Here's how the part is built. I have some questions about the finished solid (model axes, mm). Face numbers are marked on the shaded views. Coordinates: 2 decimals unless noted, no trailing zeros. Loops run counter-clockwise (first coordinate to the right, second up) from the corner with the lowest first, then second, coordinate; pieces in that order, holes last. Notation, with made-up numbers: M 70.5,-8.75 L 122.5,-8.75 A35 cw 122.5,30.25 Z; hole C 77,46.5 d10. An arc over 180 degrees is marked long. Use CSV: the item, a comma, the result in double quotes. Start each with the question number.
Q1. If we section it at B-B (x = -2.5): Please give me the cut outline in (y, z) (3 decimals), and give its area (3 significant figures).
Q2. Please list where these lines run through material, in increasing order: probe 1 along Y at (x, z) = (15, 1) (3 decimals); probe 2 along Y at (x, z) = (14.5, 2.05) (3 decimals); probe 3 along Y at (x, z) = (21, 3.55). Write a range as [from, to].
Q3. If we mould it in two halves opening along Y, with no side actions, what happens to the marked faces 1, 2 and 3? For each: +Y half, -Y half, draft (parallel to the pull), parting line (faces both ways), or undercut.
Q4. If we section it at C-C (z = 0.4): State how many separate pieces and enclosed holes the cut face has, and give its area (3 significant figures).
Q5. For pin 1 Ø1.8 at (y, z) = (8.5, 2.5) entering from -X; pin 2 Ø2 at (x, z) = (4.5, 2.5) entering from -Y, each with a flat end and sliding along its axis, tell me the tip position at first contact or that it passes through.
Q6. If we section it at A-A (y = 21): Please give me the cut outline in (x, z) (3 decimals).
Q7. If we section it at D-D (x = 14.5): Please give me the cut outline in (y, z) (3 decimals), and give its area (3 significant figures).
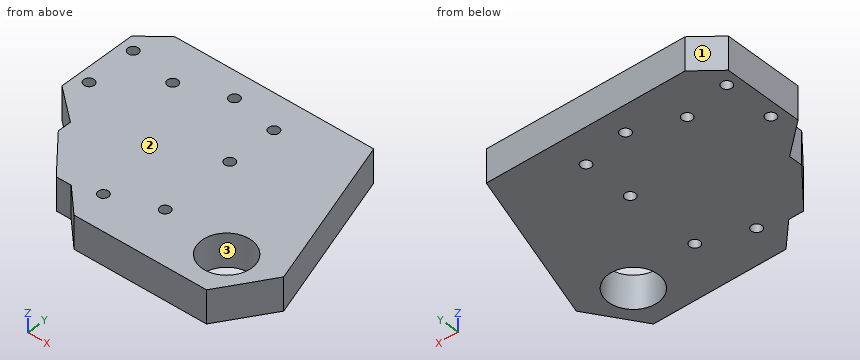
from build123d import *

# Parameters (mm, degrees)
SKETCH_1_R               = 3
EXTRUDE_1_DEPTH          = 4
HOLE_WIZARD_M1_6_1_D     = 1.25
HOLE_WIZARD_M1_6_1_DEPTH = 4.95
HOLE_WIZARD_M1_6_1_TIP   = 0.375537887
HOLE_WIZARD_M1_6_2_D     = 1.25
HOLE_WIZARD_M1_6_2_DEPTH = 4.95
HOLE_WIZARD_M1_6_2_TIP   = 0.375537887
CHAMFER_1_SIZE           = 5
CHAMFER_1_SIZE2          = 4.195498156
CHAMFER_2_SIZE2          = 4
CHAMFER_2_SIZE           = 3.356398525
CHAMFER_4_SIZE           = 3
CHAMFER_4_SIZE2          = 2.517298894


with BuildPart() as part:
    # 草图1 → 凸台-拉伸1 (new body)
    with BuildSketch(Plane.XY):
        Polygon((0, 3), (0, 13), (-4, 13), (-4, 25), (23, 25), (29, 6), (25, 0), (9, 0), (6, 3), align=None)
        with Locations((23, 5)):
            Circle(SKETCH_1_R, mode=Mode.SUBTRACT)
    extrude(amount=EXTRUDE_1_DEPTH)

    # M1.6 螺纹孔1
    with Locations(Plane.XY.offset(4)):
        with Locations((-2.5, 21), (14.5, 21), (14.5, 15), (-2.5, 15)):
            Hole(HOLE_WIZARD_M1_6_1_D / 2, depth=HOLE_WIZARD_M1_6_1_DEPTH)
            with Locations((0, 0, -(HOLE_WIZARD_M1_6_1_DEPTH + HOLE_WIZARD_M1_6_1_TIP / 2))):  # 118° drill point
                Cone(0, HOLE_WIZARD_M1_6_1_D / 2, HOLE_WIZARD_M1_6_1_TIP, mode=Mode.SUBTRACT)

    # M1.6 螺纹孔2
    with Locations(Plane.XY.offset(4)):
        with Locations((8.823813288, 22.026895413), (14.638155725, 6.05212086), (9, 4), (3.185657563, 19.974774553)):
            Hole(HOLE_WIZARD_M1_6_2_D / 2, depth=HOLE_WIZARD_M1_6_2_DEPTH)
            with Locations((0, 0, -(HOLE_WIZARD_M1_6_2_DEPTH + HOLE_WIZARD_M1_6_2_TIP / 2))):  # 118° drill point
                Cone(0, HOLE_WIZARD_M1_6_2_D / 2, HOLE_WIZARD_M1_6_2_TIP, mode=Mode.SUBTRACT)

    # 倒角1
    chamfer_1_edges = [part.edges().sort_by_distance(p)[0] for p in [
        (0, 3, 2),
    ]]
    chamfer_1_side = [part.faces().sort_by_distance(p)[0] for p in [
        (0, 8, 2),
    ]]
    chamfer(chamfer_1_edges, length=CHAMFER_1_SIZE, length2=CHAMFER_1_SIZE2, reference=chamfer_1_side[0])

    # 倒角2
    chamfer_2_edges = [part.edges().sort_by_distance(p)[0] for p in [
        (0, 13, 2),
    ]]
    chamfer_2_side = [part.faces().sort_by_distance(p)[0] for p in [
        (0, 12.93287203, 2),
    ]]
    chamfer(chamfer_2_edges, length=CHAMFER_2_SIZE - 0.0001, length2=CHAMFER_2_SIZE2 - 0.0001, reference=chamfer_2_side[0])  # a hair under: the kernel refuses the full size

    # 倒角4
    chamfer_4_edges = [part.edges().sort_by_distance(p)[0] for p in [
        (-4, 25, 2),
    ]]
    chamfer_4_side = [part.faces().sort_by_distance(p)[0] for p in [
        (9.5, 25, 2),
    ]]
    chamfer(chamfer_4_edges, length=CHAMFER_4_SIZE, length2=CHAMFER_4_SIZE2, reference=chamfer_4_side[0])


solid = part.part
Results below:
1,outline,"M 11.741,0 L 14.375,0 L 14.375,4 L 11.741,4 Z; M 15.625,0 L 20.375,0 L 20.375,4 L 15.625,4 Z; M 21.625,0 L 23.741,0 L 23.741,4 L 21.625,4 Z"
1,area,"38.0 mm^2"
2,probe 1,"[0, 5.543], [6.562, 14.625], [15.375, 20.625], [21.375, 25]"
2,probe 2,"[0, 5.443], [6.662, 14.375], [15.625, 20.375], [21.625, 25]"
2,probe 3,"[0, 2.76], [7.24, 25]"
3,face 1,"+Y half"
3,face 2,"draft"
3,face 3,"undercut"
4,separate pieces,"1"
4,enclosed holes,"9"
4,area,"636 mm^2"
5,pin 1,"x = 0"
5,pin 2,"y = 3"
6,outline,"M -4,0 L -3.125,0 L -3.125,4 L -4,4 Z; M -1.875,0 L 13.875,0 L 13.875,4 L -1.875,4 Z; M 15.125,0 L 24.263,0 L 24.263,4 L 15.125,4 Z"
7,outline,"M 0,0 L 5.443,0 L 5.443,4 L 0,4 Z; M 6.662,0 L 14.375,0 L 14.375,4 L 6.662,4 Z; M 15.625,0 L 20.375,0 L 20.375,4 L 15.625,4 Z; M 21.625,0 L 25,0 L 25,4 L 21.625,4 Z"
7,area,"85.1 mm^2"
